```python
from build123d import *

# Parameters (mm, degrees)
BOSS_EXTRUDE1_DEPTH = 5
SKETCH3_R           = 3.8
CUT_EXTRUDE1_DEPTH  = 6


with BuildPart() as part:
    # Sketch2 → Boss-Extrude1 (new body)
    with BuildSketch(Plane(origin=(0, 0, 0), x_dir=(1, 0, 0), z_dir=(0, 1, 0))):
        Polygon((0, -13.7), (39.336112578, -13.7), (64.132518911, -21.5), (144.132518911, -21.5), (165, -6), (200, -6), (200, 6), (165, 6), (144.132518911, 21.5), (64.132518911, 21.5), (39.336112578, 13.7), (0, 13.7), (0, 7.2), (35, 7.2), (35, -7.2), (0, -7.2), align=None)
    extrude(amount=BOSS_EXTRUDE1_DEPTH)

    # Sketch3 → Cut-Extrude1 (cut, through all)
    with BuildSketch(Plane(origin=(0, 5, 0), x_dir=(1, 0, 0), z_dir=(0, 1, 0))):
        with Locations((193, 0)):
            Circle(SKETCH3_R)
        Polygon((41, 7.409395112), (41, -7.409395112), (65.130733731, -15), (141.982577641, -15), (162.176914179, 0), (141.982577641, 15), (65.130733731, 15), align=None)
    extrude(amount=-CUT_EXTRUDE1_DEPTH, mode=Mode.SUBTRACT)


solid = part.part
```
Here's how the part is built. I have some questions about the finished solid (model axes, mm). A direction names the side the tool comes from. Round coordinates to 2 decimals unless told otherwise and drop trailing zeros. Loops run counter-clockwise (first coordinate to the right, second up) from the corner with the lowest first, then second, coordinate; pieces in that order, holes last. Notation, with made-up numbers: (-20, -32.5) -> (27, -32.5) arc R14 cw to (27, -27.5) -> close; hole circle Ø2 at (63, 46.5). An arc over 180 degrees is marked (long way). Answer as CSV lines item,"result". Start each with the question number.
1. I need wall thicknesses on probe 1 along X at (y, z) = (4.4, 0); probe 2 along Z at (x, y) = (193, 2.8); probe 3 along Z at (x, y) = (110, 1.6). Which ranges of each line are inside material? Lowest first, please. Write a range as from..to.
2. Imagine slicing it at B-B on y = 3.8. Write out the boundary of the cut face in (x, z), plus the area to 3 significant figures.
3. If we mould it in two halves opening along Z, with no side actions, what happens to faces 4 (the face through (104, 2, 21.5)), 5 (the face through (52.896, 2.535, 11.152)), 6 (the face through (183, 2, -6)), 7 (the face through (0, 2, 10))? For each: pulls with the +Z half, pulls with the -Z half, needs draft (parallel to the pull), parting line crosses it, or undercut.
4. Imagine slicing it at D-D on x = 172. Write out the boundary of the cut face in (y, z), plus the area to 3 significant figures.
5. I'm going to push flat-ended pins straight in: P1, Ø2, axis at x = 40, y = 1, coming from the +Z side; P2, Ø2.5, axis at x = 24, y = 2.5, coming from the +Z side; P3, Ø1, axis at x = 158.5, z = 13, coming from the +Y side; P4, Ø2.5, axis at x = 174, y = 2, coming from the -Z side. Where does each tip first touch, or does it pass through?
6. Imagine slicing it at C-C on z = 11. Write out the boundary of the cut face in (x, y).
7. For faces 1 (the face through (20, 2, -13.7)), 2 (the face through (152.221, 2.535, -7.395)), 3 (the face through (17, 2, -7.2)), which set-ups out of +Z, -Z, +X, -X, +Y, -Y let a thin tool reach every point of the face, with its end or its side?
8. Imagine slicing it at A-A on x = 93. Write out the boundary of the cut face in (y, z).
Solution:
1,probe 1,"35..41, 162.18..189.2, 196.8..200"
1,probe 2,"-6..-3.8, 3.8..6"
1,probe 3,"-21.5..-15, 15..21.5"
2,outline,"(0, -13.7) -> (39.34, -13.7) -> (64.13, -21.5) -> (144.13, -21.5) -> (165, -6) -> (200, -6) -> (200, 6) -> (165, 6) -> (144.13, 21.5) -> (64.13, 21.5) -> (39.34, 13.7) -> (0, 13.7) -> (0, 7.2) -> (35, 7.2) -> (35, -7.2) -> (0, -7.2) -> close; hole (41, -7.41) -> (65.13, -15) -> (141.98, -15) -> (162.18, 0) -> (141.98, 15) -> (65.13, 15) -> (41, 7.41) -> close; hole circle Ø7.6 at (193, 0)"
2,area,"2,690 mm²"
3,face 4,"pulls with the +Z half"
3,face 5,"undercut"
3,face 6,"pulls with the -Z half"
3,face 7,"needs draft"
4,outline,"(0, -6) -> (5, -6) -> (5, 6) -> (0, 6) -> close"
4,area,"60.0 mm²"
5,P1,"z = 14.22"
5,P2,"z = 13.7"
5,P3,"through"
5,P4,"z = -6"
6,outline,"(0, 0) -> (52.41, 0) -> (52.41, 5) -> (0, 5) -> close; (147.37, 0) -> (158.27, 0) -> (158.27, 5) -> (147.37, 5) -> close"
7,face 1,"-Z, -X, +Y, -Y"
7,face 2,"+Y, -Y"
7,face 3,"-X, +Y, -Y"
8,outline,"(0, -21.5) -> (5, -21.5) -> (5, -15) -> (0, -15) -> close; (0, 15) -> (5, 15) -> (5, 21.5) -> (0, 21.5) -> close"
